Work out the finished part from the listing and answer in its coordinate system (mm). A direction names the side the tool comes from. Round coordinates to 2 decimals unless told otherwise and drop trailing zeros. Write each loop counter-clockwise with the first axis right and the second up, starting at its lowest first coordinate (ties: lowest second). Pieces come first, ordered by that corner, then holes. Notation, with made-up numbers: (64.25, 60.25) - (73.25, 60.25) arc R30 cw to (73.25, 92.25) - close; hole circle Ø4 at (-38.75, -17). An arc over 180 degrees is marked (long way). Answer as a JSON object with one key per item and string values.
Autodesk Inventor part; units mm, degrees
ref_plane "YZ Plane" through (0, 0, 0) normal (1, 0, 0) x (0, 1, 0)
ref_plane "XZ Plane" through (0, 0, 0) normal (0, 1, 0) x (-1, 0, 0)
ref_plane "XY Plane" through (0, 0, 0) normal (0, 0, 1) x (1, 0, 0)
sketch "Skizze1" plane through (0, 0, 0) normal (0, 1, 0) x (-1, 0, 0)
  line L0 (0, 0) -> (4, 0)
  line L1 (4, 0) -> (4, -8)
  line L2 (4, -8) -> (6, -8)
  line L3 (6, -8) -> (6, -40)
  line L4 (6, -40) -> (4, -40)
  line L5 (4, -40) -> (4, -48)
  line L6 (4, -48) -> (0, -48)
  line L7 (0, -48) -> (0, 0)
  dimension "d0" = 8
  dimension "d1" = 32
  dimension "d2" = 8
  dimension "d3" = 8
  dimension "d4" = 12
revolve "Umdrehung1" add sketch "Skizze1" angle 360 about axis through (0, 0, -48) along (0, 0, 1)
thread "Gewinde1"
equation "\"d2\" = d0"
properties part number "17"
Item 1: A cutting plane is placed at C-C (z = -17). Write down the section's boundary in (x, y), and give its area (3 significant figures).
Results found:
{"outline": "circle Ø12 at (0, 0)", "area": "113 mm²"}
Item 2: Consider line 1 along Z through (x, y) = (-4.25, -1.5); line 2 along Y through (x, z) = (5.5, -13); line 3 along Y through (x, z) = (-4, -20.5). Determine where each line is inside the solid, lowest interval first.
Results found:
{"line 1": "-40 to -8", "line 2": "-2.4 to 2.4", "line 3": "-4.47 to 4.47"}
Item 3: For faces 1 (the flat face through (1.42, 3.92, -8)), 2 (the cylindrical face through (0.867, -3.905, -44.056)), 3 (the cylindrical face through (6, 0, -24)), determine the directions among +Z, -Z, +X, -X, +Y, -Y from which every point of the face is accessible in a straight line to the end or side of a thin tool.
Results found:
{"face 1": "+Z", "face 2": "-Z", "face 3": "+Z, -Z"}
Item 4: Each of these flat-tipped pins is pushed along its axis until it touches: P1, Ø1.5, axis at y = -2, z = -25.5, coming from the -X side; P2, Ø4, axis at y = 4, z = -12, coming from the -X side; P3, Ø1.5, axis at y = 3.5, z = -35, coming from the -X side. Where does it stop, or does it pass through?
Results found:
{"P1": "x = -5.87", "P2": "x = -5.66", "P3": "x = -5.33"}
Item 5: A cutting plane is placed at A-A (y = 0). Write down the section's boundary in (x, z).
Results found:
{"outline": "(-6, -40) - (-4, -40) - (-4, -48) - (4, -48) - (4, -40) - (6, -40) - (6, -8) - (4, -8) - (4, 0) - (-4, 0) - (-4, -8) - (-6, -8) - close"}
Item 6: A cutting plane is placed at D-D (x = 5). Write down the section's boundary in (y, z).
Results found:
{"outline": "(-3.32, -40) - (3.32, -40) - (3.32, -8) - (-3.32, -8) - close"}
